Verification items for the finished model (mm, model axes). A direction names the side the tool comes from. Round coordinates to 2 decimals unless told otherwise and drop trailing zeros. Return JSON: item names as keys, results as strings. Group by question number.
from build123d import *

# Parameters (mm, degrees)
SKETCH1_R                   = 30
SKETCH1_R_2                 = 2
BOSS_EXTRUDE2_DEPTH         = 5
SKETCH2_R                   = 0.15
CUT_EXTRUDE1_DEPTH          = 43.720018727
LPATTERN1_COUNT             = 4
LPATTERN1_PITCH             = 1
CIRPATTERN1_COUNT           = 4
CIRPATTERN1_COPY_1_SKETCH_R = 0.15
CIRPATTERN1_COPY_1_DEPTH    = 43.720018727
CIRPATTERN1_COPY_2_SKETCH_R = 0.15
CIRPATTERN1_COPY_2_DEPTH    = 43.720018727
CIRPATTERN1_COPY_3_SKETCH_R = 0.15
CIRPATTERN1_COPY_3_DEPTH    = 43.720018727
CIRPATTERN1_COPY_4_SKETCH_R = 0.15
CIRPATTERN1_COPY_4_DEPTH    = 43.720018727
CIRPATTERN1_COPY_5_SKETCH_R = 0.15
CIRPATTERN1_COPY_5_DEPTH    = 43.720018727
CIRPATTERN1_COPY_6_SKETCH_R = 0.15
CIRPATTERN1_COPY_6_DEPTH    = 43.720018727
CIRPATTERN1_COPY_7_SKETCH_R = 0.15
CIRPATTERN1_COPY_7_DEPTH    = 43.720018727
CIRPATTERN1_COPY_8_SKETCH_R = 0.15
CIRPATTERN1_COPY_8_DEPTH    = 43.720018727
CIRPATTERN1_COPY_9_SKETCH_R = 0.15
CIRPATTERN1_COPY_9_DEPTH    = 43.720018727
BOSS_EXTRUDE3_DEPTH         = 5
CIRPATTERN2_COUNT           = 30


with BuildPart() as part:
    # Sketch1 → Boss-Extrude2 (new body)
    with BuildSketch(Plane(origin=(0, 0, 0), x_dir=(0, 0, -1), z_dir=(1, 0, 0))):
        Circle(SKETCH1_R)
        Circle(SKETCH1_R_2, mode=Mode.SUBTRACT)
    extrude(amount=BOSS_EXTRUDE2_DEPTH)

    # Sketch2 → Cut-Extrude1 (cut, through all)
    with BuildSketch(Plane(origin=(5, 0, 0), x_dir=(0, 0, -1), z_dir=(1, 0, 0))):
        with Locations((0, 5)):
            Circle(SKETCH2_R)
    cut_extrude1 = extrude(amount=-CUT_EXTRUDE1_DEPTH, mode=Mode.SUBTRACT)

    # LPattern1: Cut-Extrude1 ×4
    with Locations(*[(0, i * LPATTERN1_PITCH, 0) for i in range(1, LPATTERN1_COUNT)]):
        add(cut_extrude1, mode=Mode.SUBTRACT)

    # CirPattern1: Cut-Extrude1 ×4 about axis
    cirpattern1_axis = Axis((0, 0, 0), (1, 0, 0))
    for i in range(1, CIRPATTERN1_COUNT):
        add(cut_extrude1.rotate(cirpattern1_axis, i * 360 / CIRPATTERN1_COUNT), mode=Mode.SUBTRACT)

    # CirPattern1 copy 1 sketch → CirPattern1 copy 1 (cut, through all)
    with BuildSketch(Plane(origin=(5, 0, 1), x_dir=(0, 1, 0), z_dir=(1, 0, 0))):
        with Locations((0, 5)):
            Circle(CIRPATTERN1_COPY_1_SKETCH_R)
    extrude(amount=-CIRPATTERN1_COPY_1_DEPTH, mode=Mode.SUBTRACT)

    # CirPattern1 copy 2 sketch → CirPattern1 copy 2 (cut, through all)
    with BuildSketch(Plane(origin=(5, -1, 0), x_dir=(0, 0, 1), z_dir=(1, 0, 0))):
        with Locations((0, 5)):
            Circle(CIRPATTERN1_COPY_2_SKETCH_R)
    extrude(amount=-CIRPATTERN1_COPY_2_DEPTH, mode=Mode.SUBTRACT)

    # CirPattern1 copy 3 sketch → CirPattern1 copy 3 (cut, through all)
    with BuildSketch(Plane(origin=(5, 0, -1), x_dir=(0, -1, 0), z_dir=(1, 0, 0))):
        with Locations((0, 5)):
            Circle(CIRPATTERN1_COPY_3_SKETCH_R)
    extrude(amount=-CIRPATTERN1_COPY_3_DEPTH, mode=Mode.SUBTRACT)

    # CirPattern1 copy 4 sketch → CirPattern1 copy 4 (cut, through all)
    with BuildSketch(Plane(origin=(5, 0, 2), x_dir=(0, 1, 0), z_dir=(1, 0, 0))):
        with Locations((0, 5)):
            Circle(CIRPATTERN1_COPY_4_SKETCH_R)
    extrude(amount=-CIRPATTERN1_COPY_4_DEPTH, mode=Mode.SUBTRACT)

    # CirPattern1 copy 5 sketch → CirPattern1 copy 5 (cut, through all)
    with BuildSketch(Plane(origin=(5, -2, 0), x_dir=(0, 0, 1), z_dir=(1, 0, 0))):
        with Locations((0, 5)):
            Circle(CIRPATTERN1_COPY_5_SKETCH_R)
    extrude(amount=-CIRPATTERN1_COPY_5_DEPTH, mode=Mode.SUBTRACT)

    # CirPattern1 copy 6 sketch → CirPattern1 copy 6 (cut, through all)
    with BuildSketch(Plane(origin=(5, 0, -2), x_dir=(0, -1, 0), z_dir=(1, 0, 0))):
        with Locations((0, 5)):
            Circle(CIRPATTERN1_COPY_6_SKETCH_R)
    extrude(amount=-CIRPATTERN1_COPY_6_DEPTH, mode=Mode.SUBTRACT)

    # CirPattern1 copy 7 sketch → CirPattern1 copy 7 (cut, through all)
    with BuildSketch(Plane(origin=(5, 0, 3), x_dir=(0, 1, 0), z_dir=(1, 0, 0))):
        with Locations((0, 5)):
            Circle(CIRPATTERN1_COPY_7_SKETCH_R)
    extrude(amount=-CIRPATTERN1_COPY_7_DEPTH, mode=Mode.SUBTRACT)

    # CirPattern1 copy 8 sketch → CirPattern1 copy 8 (cut, through all)
    with BuildSketch(Plane(origin=(5, -3, 0), x_dir=(0, 0, 1), z_dir=(1, 0, 0))):
        with Locations((0, 5)):
            Circle(CIRPATTERN1_COPY_8_SKETCH_R)
    extrude(amount=-CIRPATTERN1_COPY_8_DEPTH, mode=Mode.SUBTRACT)

    # CirPattern1 copy 9 sketch → CirPattern1 copy 9 (cut, through all)
    with BuildSketch(Plane(origin=(5, 0, -3), x_dir=(0, -1, 0), z_dir=(1, 0, 0))):
        with Locations((0, 5)):
            Circle(CIRPATTERN1_COPY_9_SKETCH_R)
    extrude(amount=-CIRPATTERN1_COPY_9_DEPTH, mode=Mode.SUBTRACT)

    # Sketch7 → Boss-Extrude3 (add)
    with BuildSketch(Plane(origin=(5, 0, 0), x_dir=(0, 0, -1), z_dir=(1, 0, 0))):
        Polygon((-1.681504774, 29.509212722), (2.818495226, 29.509212722), (1.362614288, 33.509212722), (-0.225623837, 33.509212722), align=None)
    boss_extrude3 = extrude(amount=-BOSS_EXTRUDE3_DEPTH)

    # CirPattern2: Boss-Extrude3 ×30 about axis
    cirpattern2_axis = Axis((0, 0, 0), (1, 0, 0))
    for i in range(1, CIRPATTERN2_COUNT):
        add(boss_extrude3.rotate(cirpattern2_axis, i * 360 / CIRPATTERN2_COUNT))


solid = part.part
1. Access from +Z, -Z, +X, -X, +Y, -Y to the whole of each face (thin tool, end or side, straight path). Record for faces 4 (the face through (2.535, 5.332, 31.283)), 5 (the face through (2.535, -30.554, 8.572)), 6 (the face through (2.465, -21.889, 20.515)).
2. Thickness scan on line 1 along Z through (x, y) = (0.45, -26); line 2 along Z through (x, y) = (3.55, 22.5); line 3 along Z through (x, y) = (0.55, -0.5). Record the ranges inside material, lowest first. Write a range as from..to.
3. Go/stop test with flat-tipped pins: pin 1 (2 mm diameter, centred on x = 3, z = -16, fed in from -Y); pin 2 (3 mm diameter, centred on x = 1, z = -17, fed in from +Y). Record where each tip stops, or that it passes through.
4. Cross-section at A-A (x = 0.95). Give the number of separate pieces and of enclosed holes in the cut face, plus the area to 3 significant figures.
5. Draft check along Z on faces 1 (the face through (2.465, -0.599, -29.994)), 2 (the face through (2.46, 28.34, -9.84)), 3 (the face through (2.535, 8.994, 30.472)). Enter one of: +Z half, -Z half, draft (parallel to the pull), parting line (faces both ways), or undercut.
Computed:
{
 "1": {"face 4": "+Z, +X, -X", "face 5": "+X, -X, -Y", "face 6": "+X, -X"},
 "2": {"line 1": "z = -19.6..-15.76, -14.97..14.97, 17.67..20.71", "line 2": "z = -24.83..-24.53, -19.84..19.84, 21.68..24.83", "line 3": "z = -30..-1.94, 1.94..30.09"},
 "3": {"pin 1": "stops at y = -26.84", "pin 2": "stops at y = 26.56"},
 "4": {"separate pieces": "1", "enclosed holes": "17", "area": "3,120 mm²"},
 "5": {"face 1": "-Z half", "face 2": "undercut", "face 3": "+Z half"}
}
